Geometry: see drawing. Coordinates: mm, zero at the bounding-box minimum. A direction names the side the tool comes from. Give positions to 0.01 mm unless a question says otherwise; leave off trailing zeros. Loops run counter-clockwise (first coordinate to the right, second up) from the corner with the lowest first, then second, coordinate; pieces in that order, holes last. Notation, with made-up numbers: M -5.75,67.25 L 31.25,67.25 A30 cw 31.25,95.25 Z; hole C 27.5,33.25 d9. An arc over 180 degrees is marked long. Use a Markdown table: item, result. Add a question column.
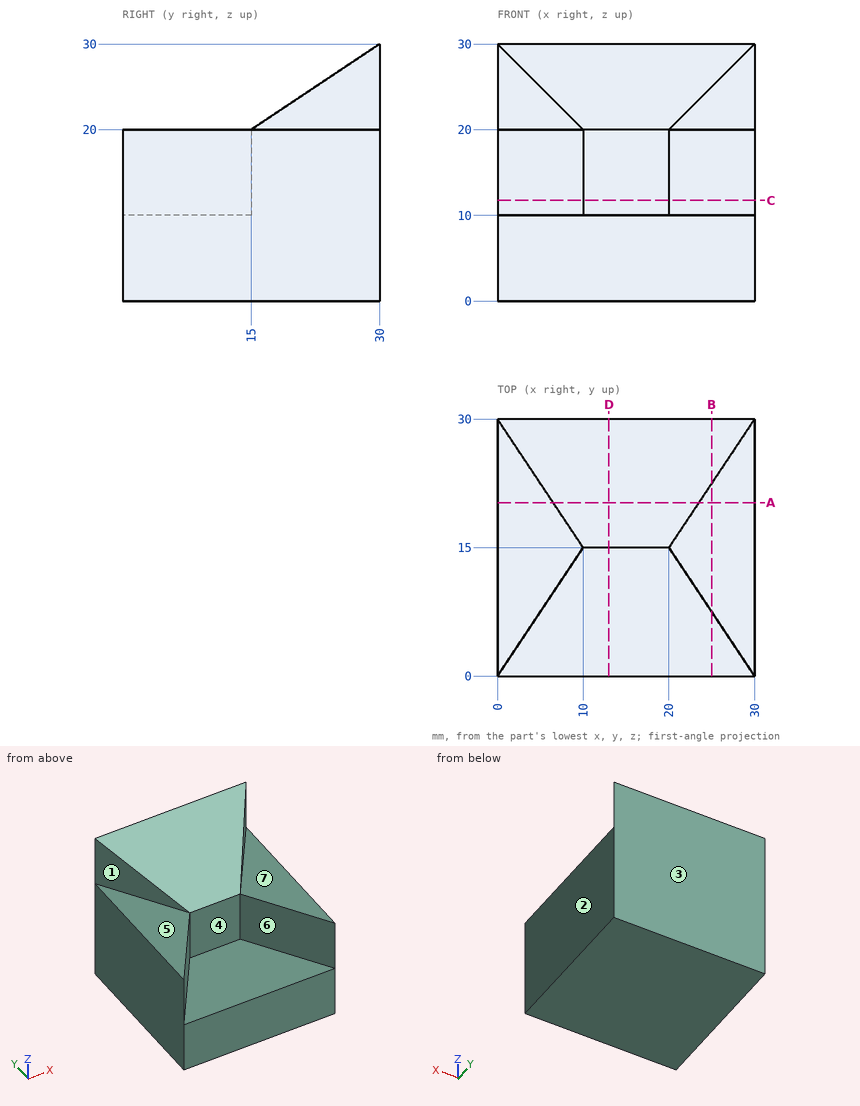
1) Section query A-A, the plane y = 20.25. Return the cut outline in (x, z), and give its area (4 significant figures).
2) Reachability of the marked faces 5, 6 and 7 from +Z, -Z, +X, -X, +Y, -Y: full face, straight path, thin tool, end or side. Return the list, or none.
3) Contact query for flat-ended pins moving along their axis: P1, Ø4, axis at x = 20, z = 16, coming from the -Y side; P2, Ø10, axis at x = 12.5, y = 19.5, coming from the +Z side; P3, Ø3, axis at x = 12, y = 18, coming from the -Z side; P4, Ø16.5, axis at x = 8.5, y = 8, coming from the +Z side. Output: stop coordinate, or through.
4) Pull-direction query (X, two-part tool) for the marked faces 1, 2, 3 and 4; classes: pulls with the +X half, pulls with the -X half, needs draft (parallel to the pull), parting line crosses it, or undercut.
5) Section query B-B, the plane x = 25. Return the cut outline in (y, z).
6) Ray query, line 1 (Z direction, x = 11.5, y = 13.75); line 2 (Z direction, x = 28.5, y = 10); line 3 (X direction, y = 3.75, z = 11.25). Return the intervals inside material, ascending. Write a range as [from, to].
7) Section query C-C, the plane z = 11.75. Return the cut outline in (x, y).
8) Section query D-D, the plane x = 13. Return the cut outline in (y, z), and give its area (3 significant figures).
Entries:
| question | item | result |
|---|---|---|
| 1 | outline | M 0,0 L 30,0 L 30,20 L 23.5,20 L 23.5,23.5 L 6.5,23.5 L 6.5,20 L 0,20 Z |
| 1 | area | 659.5 mm² |
| 2 | face 5 | +Z, -X, -Y |
| 2 | face 6 | +Z, -Y |
| 2 | face 7 | +Z, +X, -Y |
| 3 | P1 | stops at y = 12 |
| 3 | P2 | stops at z = 26.33 |
| 3 | P3 | stops at z = 0 |
| 3 | P4 | stops at z = 20.81 |
| 4 | face 1 | pulls with the -X half |
| 4 | face 2 | pulls with the +X half |
| 4 | face 3 | needs draft |
| 4 | face 4 | undercut |
| 5 | outline | M 0,0 L 30,0 L 30,30 L 22.5,25 L 22.5,20 L 7.5,20 L 7.5,10 L 0,10 Z |
| 6 | line 1 | z = [0, 10] |
| 6 | line 2 | z = [0, 20] |
| 6 | line 3 | x = [0, 2.5], [27.5, 30] |
| 7 | outline | M 0,0 L 10,15 L 20,15 L 30,0 L 30,30 L 0,30 Z |
| 8 | outline | M 0,0 L 30,0 L 30,30 L 15,20 L 15,10 L 0,10 Z |
| 8 | area | 525 mm² |
